Input: dimensioned drawing with shaded views. Units: mm. Origin: part minimum x, y, z. Give positions to 0.01 mm unless a question says otherwise; leave off trailing zeros. Order: outer loops, then holes, each group sorted by start corner. A loop starts at its lowest first (then second) coordinate and runs counter-clockwise, first axis right, second up. Notation, with made-up numbers: M 16.25,83 L 69.25,83 A16 ccw 69.25,91 Z; hole C 74.25,9.5 d2. An arc over 180 degrees is marked long. Answer in a Markdown table with one row per item. Add a question column.
(1) Section query D-D, the plane x = 7.5. Return loops of the section in (y, z), plus the area to 3 significant figures.
(2) Material intervals for line 1 along X through (y, z) = (4.5, 30); line 2 along Z through (x, y) = (68.6, 4.5); line 3 along X through (y, z) = (3.75, 6.4), sorted ascending.
(3) Section query A-A, the plane z = 6.4. Return loops of the section in (x, y), plus the area to 3 significant figures.
(4) Pin query (flat end, axial travel): P1, Ø3, axis at x = 21.4, z = 6.4, coming from the -Y side. Return the tip coordinate at first contact, or that it passes through.
(5) Section query B-B, the plane x = 68.6. Return loops of the section in (y, z), plus the area to 3 significant figures.
(6) Section query C-C, the plane y = 1. Count the separate pieces of the cut face and the enclosed holes in it, plus the area to 3 significant figures.
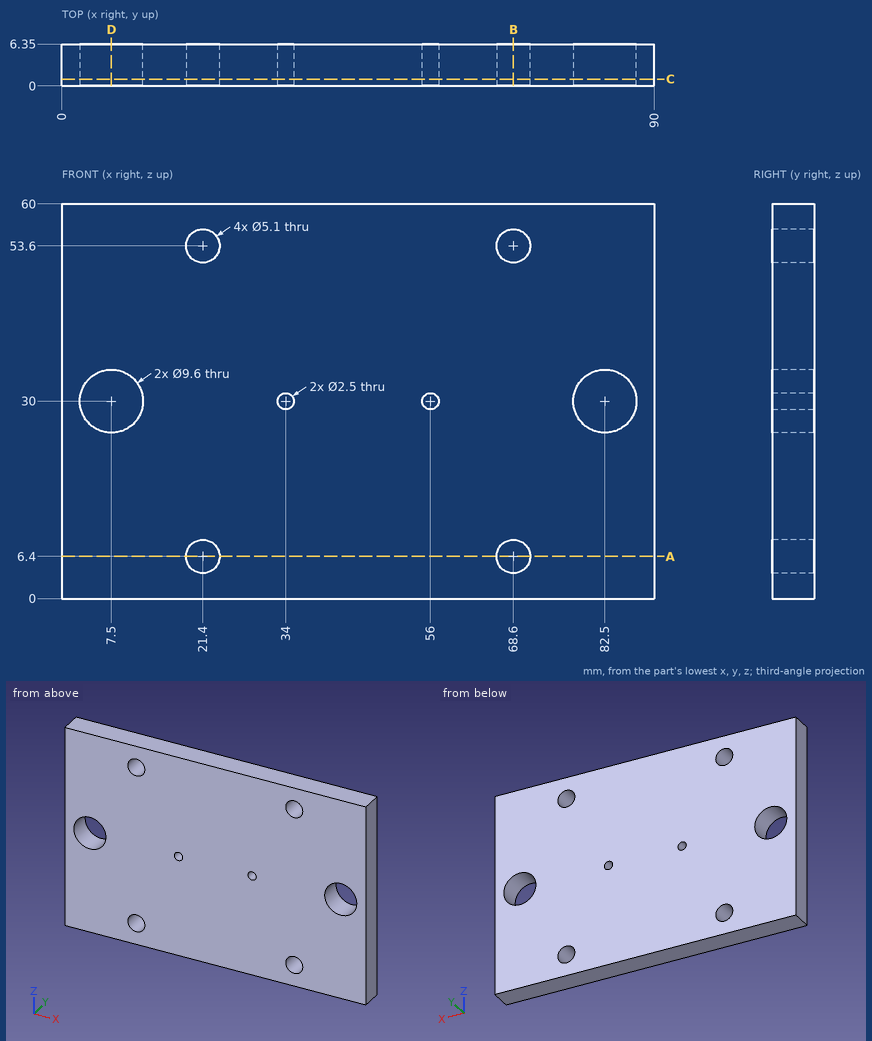
Values follow:
| question | item | result |
|---|---|---|
| 1 | outline | M 0,0 L 6.35,0 L 6.35,25.2 L 0,25.2 Z; M 0,34.8 L 6.35,34.8 L 6.35,60 L 0,60 Z |
| 1 | area | 320 mm² |
| 2 | line 1 | x = 0 to 2.7, 12.3 to 32.75, 35.25 to 54.75, 57.25 to 77.7, 87.3 to 90 |
| 2 | line 2 | z = 0 to 3.85, 8.95 to 51.05, 56.15 to 60 |
| 2 | line 3 | x = 0 to 18.85, 23.95 to 66.05, 71.15 to 90 |
| 3 | outline | M 0,0 L 18.85,0 L 18.85,6.35 L 0,6.35 Z; M 23.95,0 L 66.05,0 L 66.05,6.35 L 23.95,6.35 Z; M 71.15,0 L 90,0 L 90,6.35 L 71.15,6.35 Z |
| 3 | area | 507 mm² |
| 4 | P1 | passes through |
| 5 | outline | M 0,0 L 6.35,0 L 6.35,3.85 L 0,3.85 Z; M 0,8.95 L 6.35,8.95 L 6.35,51.05 L 0,51.05 Z; M 0,56.15 L 6.35,56.15 L 6.35,60 L 0,60 Z |
| 5 | area | 316 mm² |
| 6 | separate pieces | 1 |
| 6 | enclosed holes | 8 |
| 6 | area | 5,160 mm² |
